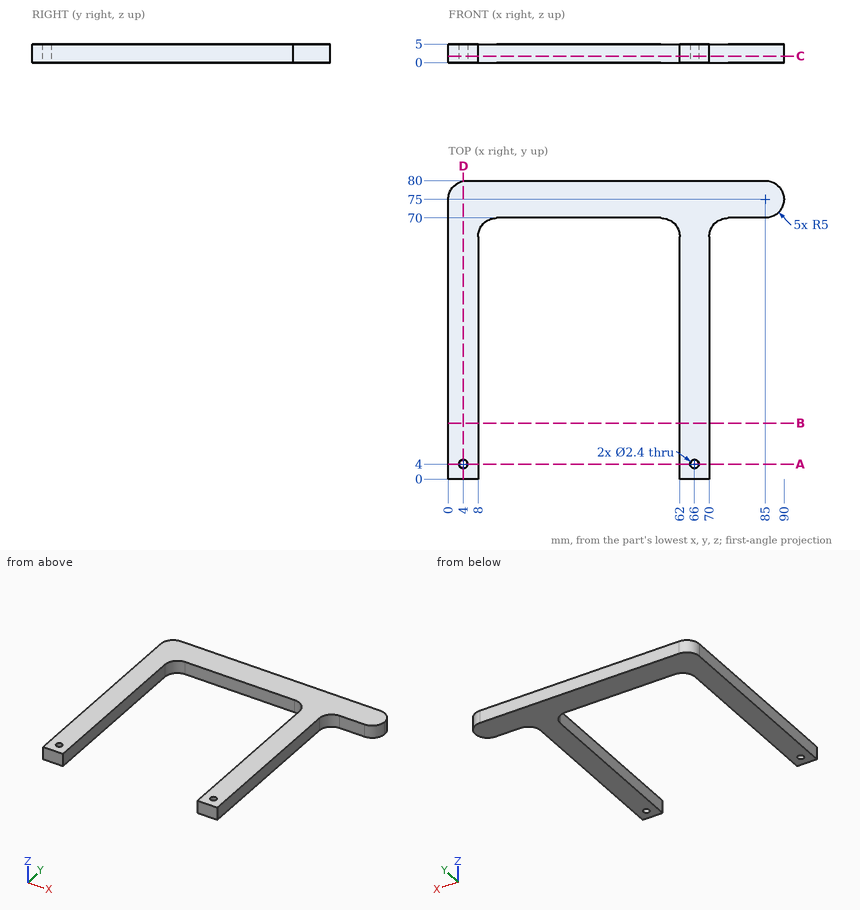
Here's the drawing with two shaded views (mm, measured from the low corner). I have some questions. Round coordinates to 2 decimals unless told otherwise and drop trailing zeros. Loops run counter-clockwise (first coordinate to the right, second up) from the corner with the lowest first, then second, coordinate; pieces in that order, holes last.
Item 1: Suppose I cut it at B-B, the plane y = 15. Write out the boundary of the cut face in (x, z).
Item 2: Please list where these lines run through material, in increasing order: L1, parallel to X at y = 4, z = 3.7; L2, parallel to X at y = 43, z = 1.15; L3, parallel to Y at x = 66, z = 1.35.
Item 3: Suppose I cut it at C-C, the plane z = 1.75. Write out the boundary of the cut face in (x, y), then the cut area to 3 significant figures.
Item 4: Suppose I cut it at D-D, the plane x = 4. Write out the boundary of the cut face in (y, z), then the cut area to 3 significant figures.
Item 5: Suppose I cut it at A-A, the plane y = 4. Write out the boundary of the cut face in (x, z).
Item 6: Will these pins go through, and if not, where does the flat tip stop? pin 1 Ø1 at (y, z) = (58.5, 2.5) entering from +X; pin 2 Ø1.5 at (x, z) = (33.5, 3) entering from -Y.
Reported:
1. outline: (0, 0) - (8, 0) - (8, 5) - (0, 5) - close; (62, 0) - (70, 0) - (70, 5) - (62, 5) - close
2. L1: x = 0 to 2.8, 5.2 to 8, 62 to 64.8, 67.2 to 70
2. L2: x = 0 to 8, 62 to 70
2. L3: y = 0 to 2.8, 5.2 to 80
3. outline: (0, 0) - (8, 0) - (8, 65) arc R5 cw to (13, 70) - (57, 70) arc R5 cw to (62, 65) - (62, 0) - (70, 0) - (70, 65) arc R5 cw to (75, 70) - (85, 70) arc R5 ccw to (85, 80) - (5, 80) arc R5 ccw to (0, 75) - close; hole circle Ø2.4 at (4, 4); hole circle Ø2.4 at (66, 4)
3. area: 2,010 mm2
4. outline: (0, 0) - (2.8, 0) - (2.8, 5) - (0, 5) - close; (5.2, 0) - (79.9, 0) - (79.9, 5) - (5.2, 5) - close
4. area: 387 mm2
5. outline: (0, 0) - (2.8, 0) - (2.8, 5) - (0, 5) - close; (5.2, 0) - (8, 0) - (8, 5) - (5.2, 5) - close; (62, 0) - (64.8, 0) - (64.8, 5) - (62, 5) - close; (67.2, 0) - (70, 0) - (70, 5) - (67.2, 5) - close
6. pin 1: stops at x = 70
6. pin 2: stops at y = 70
